CAD build for the part. Positions are in the model's coordinates, mm. A direction names the side the tool comes from. Give positions to 0.01 mm unless a question says otherwise; leave off trailing zeros. Loops run counter-clockwise (first coordinate to the right, second up) from the corner with the lowest first, then second, coordinate; pieces in that order, holes last.
Item 1: Mould opens along X. For faces 1 (the flat face through (2.921, -9, 3)), 2 (the cylindrical face through (-1.487, -6.695, 3.757)), 3 (the cylindrical face through (-0.265, -12.683, 3.131)), 4 (the cylindrical face through (0.06, -13.59, 3.13)) say: released by +X, released by -X, zero draft, split by the parting line, or undercut.
Item 2: Saw through at A-A on y = 0. Give the cut face in (x, z), plus the area to 3 significant figures.
Item 3: Saw through at C-C on z = 2.5. Give the cut face in (x, y).
Item 4: Drop flat-ended pins along their axis: P1, Ø3.5, axis at y = -9, z = 3.5, coming from the +X side; P2, Ø1.5, axis at y = -10, z = 5, coming from the +X side; P3, Ø1, axis at y = 6, z = 2, coming from the -X side. Give the stop position or say it passes through.
Item 5: Saw through at B-B on x = 0. Give the cut face in (y, z).
Item 6: Which spindle directions (+Z, -Z, +X, -X, +Y, -Y) get a long thin tool onto all of the face, cutting with end or side? Do faces 5 (the flat face through (-2.921, -9, 3)), 6 (the flat face through (2, -7, 0)). Say none if no direction does.
Item 7: Probe probe 1 along Y at (x, z) = (0, 2.75); probe 2 along X at (y, z) = (0, 3.25); probe 3 along Y at (x, z) = (-1.5, 6). List the from-to ranges inside material, lowest first.
from build123d import *

# Parameters (mm, degrees)
F0_R     = 8.001
F0_R_2   = 6.858
F1_DEPTH = 7.747
F3_R     = 2.032
F4_DEPTH = 6.35


# Not quite as in the source:
# - a fillet or chamfer that OpenCascade refuses, or shapes differently, is made with other operations: its cross-section is extruded or revolved along the edge and cut away or added


with BuildPart() as f1:
    # F0 (on Top) → F1 (new body)
    with BuildSketch(Plane.XY):
        Circle(F0_R)
        Circle(F0_R_2, mode=Mode.SUBTRACT)
    extrude(amount=F1_DEPTH)

    # F2: chamfer of 1.27 on 1 edges, made by hand

    # F2_s1 → F2_t2 (revolve, cut)
    with BuildSketch(Plane.XZ):
        Polygon((8.001, 6.477), (6.731, 7.747), (8.001, 7.747), align=None)
    revolve(axis=Axis((0, 0, 7.747), (0, 0, 1)), mode=Mode.SUBTRACT)

    # F3 (on face) → F4 (join)
    with BuildSketch(Plane(origin=(0, 0, 0), x_dir=(1, 0, 0), z_dir=(0, 0, -1))):
        with BuildLine():
            Line((2.921, 7.4487421757), (2.921, 10.668))
            ThreePointArc((2.921, 10.668), (0, 13.589), (-2.921, 10.668))
            Line((-2.921, 10.668), (-2.921, 7.4487421757))
            ThreePointArc((-2.921, 7.4487421757), (0, 8.001), (2.921, 7.4487421757))
        make_face()
        with Locations((0, 10.668)):
            Circle(F3_R, mode=Mode.SUBTRACT)
    extrude(amount=-F4_DEPTH)


solid = f1.part
Results below:
1. face 1: released by +X
1. face 2: undercut
1. face 3: undercut
1. face 4: split by the parting line
2. outline: (-8, 0) - (-6.86, 0) - (-6.86, 7.62) - (-8, 6.48) - close; (6.86, 0) - (8, 0) - (8, 6.48) - (6.86, 7.62) - close
2. area: 16.1 mm2
3. outline: (-2.92, -10.67) arc R2.92 ccw to (2.92, -10.67) - (2.92, -7.45) arc R8 ccw (long way) to (-2.92, -7.45) - close; hole circle Ø13.72 at (0, 0); hole circle Ø4.06 at (0, -10.67)
4. P1: stops at x = 3.38
4. P2: stops at x = 2.92
4. P3: stops at x = -5.81
5. outline: (-13.59, 0) - (-12.7, 0) - (-12.7, 6.35) - (-13.59, 6.35) - close; (-8.64, 0) - (-6.86, 0) - (-6.86, 7.62) - (-8, 6.48) - (-8, 6.35) - (-8.64, 6.35) - close; (6.86, 0) - (8, 0) - (8, 6.48) - (6.86, 7.62) - close
6. face 5: +Z, -Z, -X, -Y
6. face 6: -Z, +X, -X, +Y, -Y
7. probe 1: y = -13.59 to -12.7, -8.64 to -6.86, 6.86 to 8
7. probe 2: x = -8 to -6.86, 6.86 to 8
7. probe 3: y = -13.17 to -12.04, -9.3 to -6.69, 6.69 to 7.86
